The model under review builds one solid part; all positions refer to its coordinate system, in mm. A direction names the side the tool comes from. Give positions to 0.01 mm unless a question says otherwise; leave off trailing zeros. Loops run counter-clockwise (first coordinate to the right, second up) from the corner with the lowest first, then second, coordinate; pieces in that order, holes last. Notation, with made-up numbers: M 42,-28.75 L 60,-28.75 A7 cw 60,-19.75 Z; hole C -11,58.5 d5. An arc over 180 degrees is marked long. Return JSON: item names as keys, results as strings.
```python
from build123d import *

# Parameters (mm, degrees)
F0_W     = 150
F0_H     = 70
F1_DEPTH = 10
F2_R     = 4.99999
F3_R     = 2.5
F4_DEPTH = 80.75
F5_T     = -1


# Not quite as in the source:
# - a fillet or chamfer is up to 0.001 mm smaller than in the source, because OpenCascade refuses the exact size


with BuildPart() as f1:
    # F0 (on Right) → F1 (new body)
    with BuildSketch(Plane.YZ):
        Rectangle(F0_W, F0_H)
    extrude(amount=F1_DEPTH)

    # F2 (radius 5 in the source; OpenCascade refuses exactly that, so slightly less here)
    f2_edges = [f1.edges().sort_by_distance(p)[0] for p in [
        (10, 0, 35),
        (0, 0, 35),
    ]]
    fillet(f2_edges, radius=F2_R)

    # F3 (on Front) → F4 (cut, symmetric)
    with BuildSketch(Plane.XZ):
        with Locations((5, 29.747851193)):
            Circle(F3_R)
    extrude(amount=F4_DEPTH, both=True, mode=Mode.SUBTRACT)

    # F5
    f5_openings = [f1.faces().sort_by_distance(p)[0] for p in [
        (5, 0, -35),
    ]]
    offset(amount=F5_T, openings=f5_openings)


solid = f1.part
```
1) Wall thickness on L1, parallel to Y at x = 7.5, z = -8; L2, parallel to X at y = -9.5, z = 1.5; L3, parallel to Z at x = 3, y = 48.5: over which ranges is each line inside the solid? List them lowest first. Write a range as from..to.
From the geometry:
{"L1": "-75..-74, 74..75", "L2": "0..1, 9..10", "L3": "26.88..28.25, 31.25..32.62, 33.46..34.58"}
2) Consider section B-B on y = 16. Count the separate pieces of the cut face and the enclosed holes in it, then the cut area to 3 significant figures.
From the geometry:
{"separate pieces": "2", "enclosed holes": "1", "area": "163 mm²"}
3) Tool access review of faces 4 (the face through (1, -1, -2)), 5 (the face through (2.203, 1.036, 32.859)), 6 (the face through (5, -75, 0)): name each direction out of +Z, -Z, +X, -X, +Y, -Y from which nothing blocks a thin tool from reaching the whole face with its end or side.
From the geometry:
{"face 4": "-Z", "face 5": "none", "face 6": "+Z, -Z, +X, -X, -Y"}
4) Insertion check: pin 1 (3 mm diameter, centred on x = 5, z = 29.75, fed in from +Y); pin 2 (2 mm diameter, centred on x = 5.5, y = -16.5, fed in from -Z); pin 3 (5 mm diameter, centred on x = 1.5, y = -56.5, fed in from +Z). Each pin has a flat end and moves straight along its axis. Give the tip position at first contact, or say it passes through.
From the geometry:
{"pin 1": "through", "pin 2": "z = 26.25", "pin 3": "z = 34.9"}
5) Consider section A-A on z = -20. Write out the cut boundary in (x, y), then the cut area to 3 significant figures.
From the geometry:
{"outline": "M 0,-75 L 10,-75 L 10,75 L 0,75 Z; hole M 1,-74 L 9,-74 L 9,74 L 1,74 Z", "area": "316 mm²"}
6) The part is to be moulded in two halves that separate along Z. For faces 1 (the face through (6.88, -1.04, 32.7)), 2 (the face through (9.4, -0.4, -35)), 3 (the face through (2, 1, 34)), say which applies: released by +Z, released by -Z, zero draft, split by the parting line, or undercut.
From the geometry:
{"face 1": "undercut", "face 2": "released by -Z", "face 3": "released by +Z"}
